Autodesk Inventor part; units mm, degrees
ref_plane "YZ Plane" through (0, 0, 0) normal (1, 0, 0) x (0, 1, 0)
ref_plane "XZ Plane" through (0, 0, 0) normal (0, 1, 0) x (-1, 0, 0)
ref_plane "XY Plane" through (0, 0, 0) normal (0, 0, 1) x (1, 0, 0)
sketch "Sketch1" plane through (0, 0, 0) normal (1, 0, 0) x (0, 1, 0)
  line L0 (-24, -4.205) -> (-24, 1)
  line L1 (-20, 5) -> (20, 5)
  line L2 (24, 1) -> (24, -4.205)
  line L3 (20, -8.205) -> (19.9, -8.205)
  line L4 (-20, -8.205) -> (-19.9, -8.205)
  line L5 (-20.15, -2.2154) -> (-20.15, 0)
  line L6 (-20.15, 0) -> (20.15, 0)
  line L7 (20.15, 0) -> (20.15, -2.2154)
  line L8 (-0.625, 5) -> (-0.625, 13)
  line L9 (-0.625, 13) -> (0.625, 13)
  line L10 (0.625, 13) -> (0.625, 5)
  line L11 (-24, 17) -> (24, 17)
  line L12 (24, 17) -> (24, 13)
  line L13 (24, 13) -> (-24, 13)
  line L14 (-24, 13) -> (-24, 17)
  arc A0 (24, 1) -> (20, 5) centre (20, 1) ccw
  arc A1 (-20, 5) -> (-24, 1) centre (-20, 1) ccw
  arc A2 (20.15, 0) -> (13.15, 0) centre (16.65, 0) ccw
  arc A3 (-13.15, 0) -> (-20.15, 0) centre (-16.65, 0) ccw
  arc A4 (20.15, -2.2154) -> (19.9, -8.205) centre (19.9, -5.205) ccw
  arc A5 (20, -8.205) -> (24, -4.205) centre (20, -4.205) ccw
  circle A6 centre (-19.9, -5.205) radius 3
  arc A7 (-24, -4.205) -> (-20, -8.205) centre (-20, -4.205) ccw
  point P0 (0, 0)
  point P1 (-24, -8.205)
  point P2 (-24, 5)
  point P3 (24, 5)
  point P4 (24, -8.205)
  point P5 (0, 5)
  point P6 (0, 0)
  point P7 (0, 13)
  point P8 (0.625, 13)
  point P9 (-0.625, 13)
  dimension "d65" = 6
  dimension "d2" = 40.3
  dimension "d10" = 48
  dimension "d11" = 5
  dimension "d13" = 1.25
  dimension "d14" = 8
  dimension "d15" = 4
  dimension "d52" = 4
  dimension "d53" = 7
  dimension "d54" = 7
  dimension "d61" = 6
  dimension "d62" = 5.205
  dimension "d63" = 0.25
  dimension "d64" = 4
  dimension "d66" = 0.25
  dimension "d67" = 4
extrude "Extrusion1" add sketch "Sketch1" along normal mid plane 40 contours L0 A1 L1 A0 L2 A5 L3 A4 L7 A2 L6 A3 L5 A6 A7 | A6 L4 | L8 L9 L10 L1 | L13 L14 L11 L12 L9
sketch "Sketch2" plane through (-20, -24, 17) normal (0, 0, 1) x (1, 0, 0)
  line L0 (0, 0) -> (40, 0)
  line L1 (40, 48) -> (40, 0)
  line L2 (0, 48) -> (40, 48)
  line L3 (0, 0) -> (0, 48)
  line L4 (20.625, 8) -> (19.375, 8)
  line L5 (19.375, 8) -> (19.375, 40)
  line L6 (19.375, 40) -> (20.625, 40)
  line L7 (20.625, 40) -> (20.625, 8)
  line L8 (20.625, 8) -> (19.375, 40) construction
  line L9 (19.375, 8) -> (20.625, 40) construction
  point P0 (20, 24)
  point P1 (20.75, 0)
  point P2 (20.75, 50)
  point P3 (19.25, 50)
  point P4 (19.25, 0)
  point P5 (20, 8)
  dimension "d16" = 1.25
  dimension "d19" = 8
extrude "Extrusion2" add sketch "Sketch2" along normal blind 8 contours L4 L5 L6 L7
sketch "Sketch3" plane through (-20, -24, 17) normal (0, 0, 1) x (1, 0, 0)
  line L0 (20.625, 40) -> (20.625, 8)
  line L1 (20.625, 8) -> (19.375, 8)
  line L2 (19.375, 8) -> (19.375, 40)
  line L3 (19.375, 40) -> (20.625, 40)
  line L4 (0, 0) -> (40, 0)
  line L5 (40, 48) -> (40, 0)
  line L6 (0, 48) -> (40, 48)
  line L7 (0, 0) -> (0, 48)
  line L8 (20.625, 8) -> (19.375, 8)
  line L9 (20, 8) -> (20, 0)
  line L10 (19.375, 40) -> (20.625, 40)
  line L11 (20, 40) -> (20, 48)
  point P0 (20, 24)
  point P1 (20, 4)
  point P2 (20, 44)
hole "Hole1" at (0, -20, 17) at (0, 20, 17) direction (0, 0, -1) diameter 4 depth 8 tip angle 118
sketch "Sketch4" plane through (-20, -24, 25) normal (0, 0, 1) x (1, 0, 0)
  line L0 (0, 8) -> (40, 8)
  line L1 (40, 8) -> (40, 40)
  line L2 (40, 40) -> (0, 40)
  line L3 (0, 40) -> (0, 8)
  line L4 (0, 8) -> (40, 40) construction
  line L5 (40, 8) -> (0, 40) construction
  line L6 (20.625, 40) -> (19.375, 40)
  line L7 (0, 0) -> (0, 48)
  point P0 (20, 24)
  point P1 (20, 40)
  point P2 (0, 24)
extrude "Extrusion3" add sketch "Sketch4" along normal blind 5
sketch "Sketch5" plane through (-20, -24, 30) normal (0, 0, 1) x (1, 0, 0)
  line L0 (40, 40) -> (0, 40)
  line L1 (0, 40) -> (0, 8)
  line L2 (0, 8) -> (40, 8)
  line L3 (40, 8) -> (40, 40)
  line L4 (5, 24) -> (35, 24)
  point P0 (20, 24)
  point P1 (20, 24)
  dimension "d29" = 5
hole "Hole2" at (-15, 0, 30) at (15, 0, 30) direction (0, 0, -1) diameter 4 depth 8 tip angle 118
sketch "Sketch6" plane through (-20, -24, 30) normal (0, 0, 1) x (1, 0, 0)
  circle A0 centre (5, 24) radius 2
  circle A1 centre (35, 24) radius 2
  line L0 (40, 40) -> (0, 40)
  line L1 (0, 40) -> (0, 8)
  line L2 (0, 8) -> (40, 8)
  line L3 (40, 8) -> (40, 40)
  line L4 (20, 11.5) -> (20, 36.5)
  point P0 (20, 24)
  point P1 (20, 24)
  point P2 (20, 24)
  dimension "d38" = 25
hole "Hole3" at (0, -12.5, 30) at (0, 12.5, 30) direction (0, 0, -1) diameter 4 depth 5
chamfer "Chamfer1" distance 15 angle 45 4 edges at (-20, -24, 15) (-20, 24, 15) (20, -24, 15) (20, 24, 15)
chamfer "Chamfer2" distance 12 angle 45 4 edges at (20, 16, 27.5) (20, -16, 27.5) (-20, -16, 27.5) (-20, 16, 27.5)
fillet "Fillet1" radius 2 6 edges at (0.625, 0, 17) (-0.625, 0, 17) (0, -0.625, 5) (0, 0.625, 5) (0, -0.625, 13) (0, 0.625, 13)
equation "\"d54\" = d53"
properties part number "MicroRail-FlextureBase" material "ABS Plastic"
Part model, mm, in its own coordinate system. A direction names the side the tool comes from. Coordinates: 2 decimals unless noted, no trailing zeros. Write each loop counter-clockwise with the first axis right and the second up, starting at its lowest first coordinate (ties: lowest second). Pieces come first, ordered by that corner, then holes.
Item 1: Which spindle directions (+Z, -Z, +X, -X, +Y, -Y) get a long thin tool onto all of the face, cutting with end or side? Do faces 4 (the face through (0, -0.625, 9)), 5 (the face through (-0.28, 22.797, 3.859)), 6 (the face through (-14, -10, 27)), 7 (the face through (8, 0, 25)). Say none if no direction does.
Item 2: Probe line 1 (Z direction, x = 11.5, y = -9.5); line 2 (Y direction, x = 0, z = 28.25); line 3 (Y direction, x = 0, z = 14.5). List the from-to ranges inside material, lowest first.
Item 3: Mould opens along X. For faces 1 (the face through (0, -24, 15)), 2 (the face through (20, 0, 27)), 3 (the face through (0, 13, 25)) say: released by +X, released by -X, zero draft, split by the parting line, or undercut.
Item 4: Slice it at A-A (y = -8). Write the cut outline in (x, z) (3 decimals).
Item 5: Pin check, flat tips, straight feed: pin 1 (2.5 mm diameter, centred on x = 15, y = 0, fed in from -Z); pin 2 (1.5 mm diameter, centred on x = -8, z = 2, fed in from +Y); pin 3 (2.5 mm diameter, centred on x = -15, y = 0, fed in from +Z). Stop position of each tip, or through.
Item 6: Slice it at C-C (y = 0). Write the cut outline in (x, z) (3 decimals), and give its area (3 significant figures).
Item 7: Slice it at D-D (z = 15.5). Write the cut outline in (x, y), and give its area (3 significant figures).
Results found:
1. face 4: +X, -X, -Y
1. face 5: +X, -X, +Y
1. face 6: +Z, -X, -Y
1. face 7: +X, +Y, -Y
2. line 1: z = 0 to 5, 13 to 17, 25 to 30
2. line 2: y = -16 to -14.5, -10.5 to 10.5, 14.5 to 16
2. line 3: y = -24 to -22, -18 to 18, 22 to 24
3. face 1: zero draft
3. face 2: released by +X
3. face 3: undercut
4. outline: (-20, 0) - (20, 0) - (20, 5) - (-20, 5) - close; (-20, 13) - (20, 13) - (20, 17) - (2.625, 17) arc R2 cw to (0.625, 19) - (0.625, 25) - (16, 25) - (16, 30) - (-16, 30) - (-16, 25) - (-0.625, 25) - (-0.625, 19) arc R2 cw to (-2.625, 17) - (-20, 17) - close
5. pin 1: stops at z = 0
5. pin 2: stops at y = 23.99
5. pin 3: stops at z = 17
6. outline: (-20, 0) - (20, 0) - (20, 17) - (2.625, 17) arc R2 cw to (0.625, 19) - (0.625, 25) - (13, 25) - (13, 30) - (-13, 30) - (-13, 25) - (-0.625, 25) - (-0.625, 19) arc R2 cw to (-2.625, 17) - (-20, 17) - close; (-20, 25) - (-17, 25) - (-17, 30) - (-20, 30) - close; (17, 25) - (20, 25) - (20, 30) - (17, 30) - close
6. area: 852 mm2
7. outline: (-20, -9) - (-5, -24) - (5, -24) - (20, -9) - (20, 9) - (5, 24) - (-5, 24) - (-20, 9) - close; hole circle Ø4 at (0, -20); hole circle Ø4 at (0, 20)
7. area: 1,440 mm2
